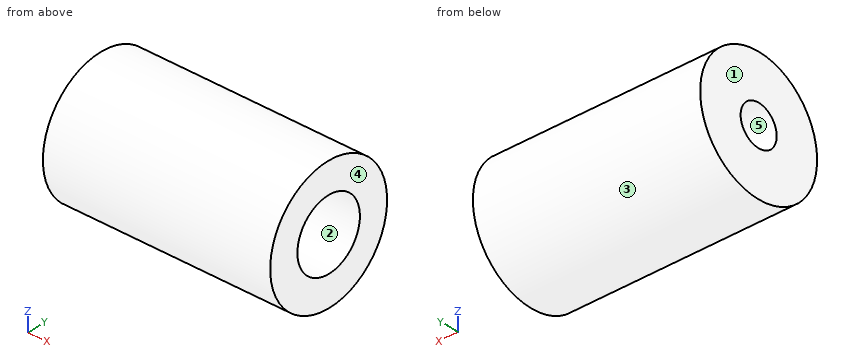
from build123d import *

# Parameters (mm, degrees)
CONN_T4_FNPT_SKETCH_W = 36
CONN_T4_FNPT_SKETCH_H = 10.287
SOCKET_1_SKETCH_W     = 15
SOCKET_1_SKETCH_H     = 5.5
SOCKET_2_SKETCH_W     = 16.2
SOCKET_2_SKETCH_H     = 3.175


with BuildPart() as part:
    # Conn_T4_FNPT Sketch → Conn_T4_FNPT (revolve)
    with BuildSketch(Plane.XY, mode=Mode.PRIVATE) as conn_t4_fnpt_sk:
        with Locations((-18, 5.1435)):
            Rectangle(CONN_T4_FNPT_SKETCH_W, CONN_T4_FNPT_SKETCH_H)
    revolve(conn_t4_fnpt_sk.sketch.rotate(Axis((-1000, 0, 0), (1, 0, 0)), 90), axis=Axis((-1000, 0, 0), (1, 0, 0)))

    # Socket 1 Sketch → Socket 1 (revolve, cut)
    with BuildSketch(Plane.XY, mode=Mode.PRIVATE) as socket_1_sk:
        with Locations((-6.5, 2.75)):
            Rectangle(SOCKET_1_SKETCH_W, SOCKET_1_SKETCH_H)
    revolve(socket_1_sk.sketch.rotate(Axis((-1000, 0, 0), (1, 0, 0)), 90), axis=Axis((-1000, 0, 0), (1, 0, 0)), mode=Mode.SUBTRACT)

    # Socket 2 Sketch → Socket 2 (revolve, cut)
    with BuildSketch(Plane.XY, mode=Mode.PRIVATE) as socket_2_sk:
        with Locations((-28.9, 1.5875)):
            Rectangle(SOCKET_2_SKETCH_W, SOCKET_2_SKETCH_H)
    revolve(socket_2_sk.sketch.rotate(Axis((-1000, 0, 0), (1, 0, 0)), 90), axis=Axis((-1000, 0, 0), (1, 0, 0)), mode=Mode.SUBTRACT)


solid = part.part
Verification items for the finished model (mm, model axes). Face numbers are marked on the shaded views. A direction names the side the tool comes from. Give positions to 0.01 mm unless a question says otherwise; leave off trailing zeros. Write each loop counter-clockwise with the first axis right and the second up, starting at its lowest first coordinate (ties: lowest second). Pieces come first, ordered by that corner, then holes.
(1) Access from +Z, -Z, +X, -X, +Y, -Y to the whole of each face (thin tool, end or side, straight path). Record for the marked faces 1 and 2.
(2) Gauge pin test, flat ends, axial feed: pin 1 (5 mm diameter, centred on y = 1, z = -1.5, fed in from -X); pin 2 (5.5 mm diameter, centred on y = 0, z = 0, fed in from -X); pin 3 (4 mm diameter, centred on x = -19.5, y = -7.5, fed in from -Z); pin 4 (12 mm diameter, centred on x = -24, z = 7, fed in from +Y). Record the tip position at first contact, or that the pin passes through.
(3) Cross-section at A-A (x = -29). Enter the section's corners in (y, z) (3 decimals).
(4) Mould release check, pull along Z, two halves, no side actions. Record for the marked faces 3, 4 and 5: +Z half, -Z half, draft (parallel to the pull), parting line (faces both ways), or undercut.
(5) Material ranges on line 1 (Y direction, x = -9, z = 0); line 2 (Y direction, x = -26.75, z = 0) (3 decimals); line 3 (X direction, y = 2.5, z = -0.5), recorded low to high.
(6) Cross-section at D-D (y = 4.5). Enter the section's corners in (x, z), plus the area to 3 significant figures.
(7) Cross-section at B-B (y = 0). Enter the section's corners in (x, z) (3 decimals).
Worked out:
1. face 1: +Z, -Z, -X, +Y, -Y
1. face 2: +X
2. pin 1: stops at x = -36
2. pin 2: stops at x = -20.8
2. pin 3: stops at z = -8.69
2. pin 4: stops at y = 10.24
3. outline: circle Ø20.574 at (0, 0); hole circle Ø6.35 at (0, 0)
4. face 3: parting line
4. face 4: draft
4. face 5: undercut
5. line 1: y = -10.29 to -5.5, 5.5 to 10.29
5. line 2: y = -10.287 to -3.175, 3.175 to 10.287
5. line 3: x = -20.8 to -14
6. outline: (-36, -9.25) - (0, -9.25) - (0, -3.16) - (-14, -3.16) - (-14, 3.16) - (0, 3.16) - (0, 9.25) - (-36, 9.25) - close
6. area: 577 mm2
7. outline: (-36, -10.287) - (0, -10.287) - (0, -5.5) - (-14, -5.5) - (-14, 5.5) - (0, 5.5) - (0, 10.287) - (-36, 10.287) - (-36, 3.175) - (-20.8, 3.175) - (-20.8, -3.175) - (-36, -3.175) - close
